Part model, mm, in its own coordinate system. Round coordinates to 2 decimals unless told otherwise and drop trailing zeros. Use a Markdown table: item, result. Add a question column.
1) Wall check: probe 1 along Z at (x, y) = (3, -51); probe 2 along X at (y, z) = (-40, 12.5); probe 3 along X at (y, z) = (-52.5, -18). Give the ranges that are in metal, low to high.
2) Slice it at A-A on y = -39.5. Give the number of separate pieces and of enclosed holes in the cut face, plus the area to 3 significant figures.
3) Drop a flat-ended pin along its axis: P1, Ø1.6, axis at x = 6, z = -18, coming from the -Y side. Give the stop position or say it passes through.
```python
from build123d import *

# Parameters (mm, degrees)
F0_W     = 70
F0_H     = 120
F1_DEPTH = 60
F2_R     = 2
F3_W     = 34
F3_H     = 30
F3_W_2   = 32
F3_H_2   = 28
F4_DEPTH = 25
F5_W     = 3
F5_H     = 4
F5_W_2   = 2
F5_H_2   = 8
F6_DEPTH = 25


with BuildPart() as f1:
    # F0 (on Front) → F1 (new body)
    with BuildSketch(Plane.XZ):
        Rectangle(F0_W, F0_H)
    extrude(amount=F1_DEPTH)

    # F2
    f2_edges = [f1.edges().sort_by_distance(p)[0] for p in [
        (35, -30, 60),
        (35, -30, -60),
        (-35, -30, 60),
        (-35, -30, -60),
        (0, -60, -60),
        (35, -60, 0),
        (0, -60, 60),
        (-35, -60, 0),
    ]]
    fillet(f2_edges, radius=F2_R)

    # F3 (on face) → F4 (cut)
    with BuildSketch(Plane.XZ.offset(60)):
        with Locations((0, 22)):
            Rectangle(F3_W, F3_H)
        with Locations((0, 22)):
            Rectangle(F3_W_2, F3_H_2, mode=Mode.SUBTRACT)
        with Locations((0, -22)):
            Rectangle(F3_W, F3_H)
        with Locations((0, -22)):
            Rectangle(F3_W_2, F3_H_2, mode=Mode.SUBTRACT)
    extrude(amount=-F4_DEPTH, mode=Mode.SUBTRACT)

    # F5 (on face) → F6 (cut)
    with BuildSketch(Plane.XZ.offset(60)):
        with Locations((0, 16)):
            Rectangle(F5_W, F5_H)
        with Locations((0, -28)):
            Rectangle(F5_W, F5_H)
        with Locations((-6, -18)):
            Rectangle(F5_W_2, F5_H_2)
        with Locations((-6, 26)):
            Rectangle(F5_W_2, F5_H_2)
        with Locations((6, 26)):
            Rectangle(F5_W_2, F5_H_2)
        with Locations((6, -18)):
            Rectangle(F5_W_2, F5_H_2)
    extrude(amount=-F6_DEPTH, mode=Mode.SUBTRACT)


solid = f1.part
```
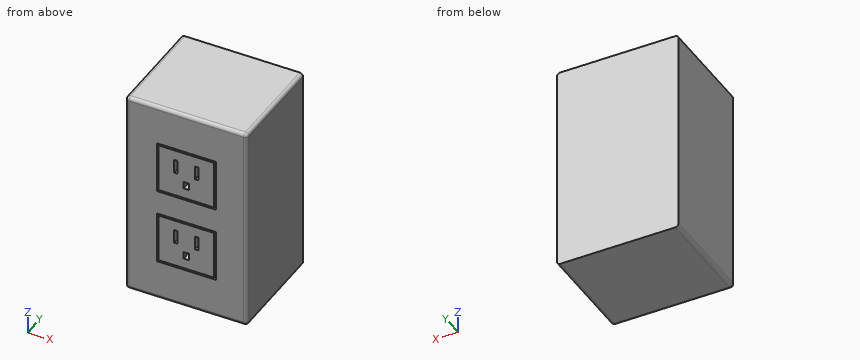
Entries:
| question | item | result |
|---|---|---|
| 1 | probe 1 | z = -60 to -37, -36 to -8, -7 to 7, 8 to 36, 37 to 60 |
| 1 | probe 2 | x = -35 to -17, -16 to 16, 17 to 35 |
| 1 | probe 3 | x = -35 to -17, -16 to -7, -5 to 5, 7 to 16, 17 to 35 |
| 2 | separate pieces | 3 |
| 2 | enclosed holes | 8 |
| 2 | area | 8,060 mm^2 |
| 3 | P1 | stops at y = -35 |
